Autodesk Inventor part; units mm, degrees
ref_plane "YZ Plane" through (0, 0, 0) normal (1, 0, 0) x (0, 1, 0)
ref_plane "XZ Plane" through (0, 0, 0) normal (0, 1, 0) x (-1, 0, 0)
ref_plane "XY Plane" through (0, 0, 0) normal (0, 0, 1) x (1, 0, 0)
sketch "スケッチ1" plane through (0, 0, 0) normal (0, 0, 1) x (1, 0, 0)
  line L0 (0, 0) -> (20, 0)
  line L1 (20, 0) -> (20, 7)
  line L2 (20, 7) -> (0, 7)
  line L3 (0, 7) -> (0, 0)
  dimension "d0" = 7
  dimension "d1" = 20
extrude "押し出し1" add sketch "スケッチ1" along normal blind 5
sketch "スケッチ2" plane through (0, 7, 0) normal (0, 1, 0) x (1, 0, 0)
  line L0 (20, 0) -> (0, 0)
  point P0 (10, -2.5)
  dimension "d4" = 2.5
hole "穴1" at (10, 7, 2.5) direction (0, -1, 0) diameter 2.459 end through all
sketch "スケッチ3" plane through (0, 0, 5) normal (0, 0, 1) x (1, 0, 0)
  line L0 (8.7705, 7) -> (11.2295, 7)
  line L1 (10, 7) -> (10, 0)
  line L2 (20, 7) -> (0, 7)
  point P0 (0, 0)
  point P1 (4, 3.5)
  point P2 (16, 3.5)
  dimension "d12" = 6
  dimension "d13" = 3.5
hole "穴2" at (4, 3.5, 5) at (16, 3.5, 5) direction (0, 0, -1) diameter 3 depth 20 tip angle 118
properties part number "シリンダーの先に着けるやつ"
Build history of the part. All positions in model axes, mm. Coordinates: 2 decimals unless noted, no trailing zeros. Write each loop counter-clockwise with the first axis right and the second up, starting at its lowest first coordinate (ties: lowest second). Pieces come first, ordered by that corner, then holes.
1. Band-saw the part on D-D, the plane z = 4.35. Give the cut face in (x, y).
Answer block:
outline: (0, 0) - (20, 0) - (20, 7) - (0, 7) - close; hole circle Ø3 at (4, 3.5); hole circle Ø3 at (16, 3.5)
2. Band-saw the part on A-A, the plane x = 10. Give the cut face in (y, z).
Answer block:
outline: (0, 0) - (7, 0) - (7, 1.27) - (0, 1.27) - close; (0, 3.73) - (7, 3.73) - (7, 5) - (0, 5) - close
3. Band-saw the part on B-B, the plane y = 3.5. Give the cut face in (x, z).
Answer block:
outline: (0, 0) - (2.5, 0) - (2.5, 5) - (0, 5) - close; (5.5, 0) - (14.5, 0) - (14.5, 5) - (5.5, 5) - close; (17.5, 0) - (20, 0) - (20, 5) - (17.5, 5) - close; hole circle Ø2.46 at (10, 2.5)
4. Band-saw the part on C-C, the plane z = 2. Give the cut face in (x, y), and give its area (3 significant figures).
Answer block:
outline: (0, 0) - (8.88, 0) - (8.88, 7) - (0, 7) - close; (11.12, 0) - (20, 0) - (20, 7) - (11.12, 7) - close; hole circle Ø3 at (4, 3.5); hole circle Ø3 at (16, 3.5)
area: 110 mm2
5. Pull direction X, two halves, no side cores. Call faces 1 (the flat face through (0, 4, 2)), 2 (the flat face through (20, 3, 2)), 3 (the flat face through (10, 4, 5)), 4 (the cylindrical face through (16, 2, 2)): released by +X, released by -X, zero draft, split by the parting line, or undercut.
Answer block:
face 1: released by -X
face 2: released by +X
face 3: zero draft
face 4: undercut
6. Drill centre lines: probe 1 along X at (y, z) = (3.5, 4.4); probe 2 along X at (y, z) = (3.5, 2.5); probe 3 along Y at (x, z) = (4, 1.6). Where is each one in solid material? Low to high.
Answer block:
probe 1: x = 0 to 2.5, 5.5 to 14.5, 17.5 to 20
probe 2: x = 0 to 2.5, 5.5 to 8.77, 11.23 to 14.5, 17.5 to 20
probe 3: y = 0 to 2, 5 to 7
